from build123d import *

# Parameters (mm, degrees)
BOSS_EXTRUDE1_DEPTH = 30


with BuildPart() as part:
    # Sketch2 → Boss-Extrude1 (new body)
    with BuildSketch(Plane(origin=(0, 0, 0), x_dir=(1, 0, 0), z_dir=(0, 1, 0))):
        with BuildLine():
            Line((0, 90), (-30, 90))
            Line((-30, 90), (-30, 87))
            Line((-30, 87), (0, 87))
            add(Edge.make_bspline(
                [(0, 87), (77.34675255, 84.211391956), (84.31600038, 0)],
                knots=[0, 0, 0, 1, 1, 1], degree=2))
            add(Edge.make_bspline(
                [(0, -87), (77.34675255, -84.211391956), (84.31600038, 0)],
                knots=[0, 0, 0, 1, 1, 1], degree=2))
            Line((0, -87), (-30, -87))
            Line((-30, -87), (-30, -90))
            Line((-30, -90), (0, -90))
            add(Edge.make_bspline(
                [(0, -90), (79.973883015, -87.051000651), (87.31600038, 0)],
                knots=[0, 0, 0, 1, 1, 1], degree=2))
            add(Edge.make_bspline(
                [(0, 90), (79.973883015, 87.051000651), (87.31600038, 0)],
                knots=[0, 0, 0, 1, 1, 1], degree=2))
        make_face()
    extrude(amount=BOSS_EXTRUDE1_DEPTH)


solid = part.part
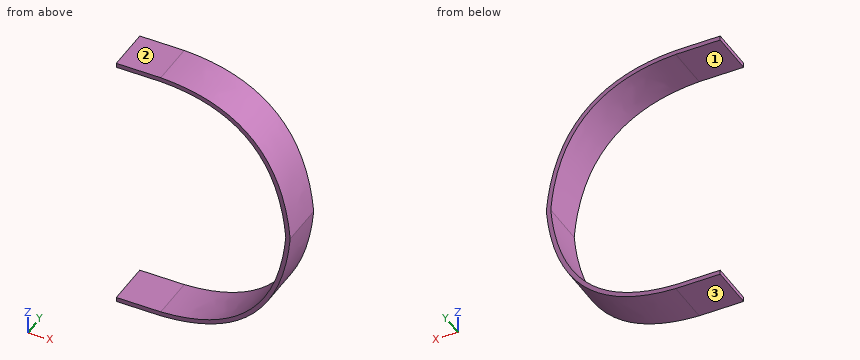
Read the model definition and answer for the solid it produces. Units are mm, in the model's axes. Face numbers are marked on the shaded views. Give positions to 0.01 mm unless a question says otherwise; leave off trailing zeros. Return JSON: item names as keys, results as strings.
Q1. Given P1, Ø10, axis at y = 8, z = 54.5, coming from the -X side; P2, Ø6, axis at x = 41, y = 18, coming from the -Z side; P3, Ø10, axis at y = 26.5, z = 53, coming from the -X side, each flat-ended and moving along its own axis, determine where each tip first touches the part or whether it passes through.
Reply:
{"P1": "x = 63.63", "P2": "z = -82.23", "P3": "x = 64.82"}
Q2. For a pull along Z with two mould halves and no side action, classify the marked faces 1, 2 and 3 as released by +Z, released by -Z, zero draft, split by the parting line, or undercut.
Reply:
{"face 1": "undercut", "face 2": "released by +Z", "face 3": "released by -Z"}
Q3. Consider line 1 along Z through (x, y) = (-11, 5.5); line 2 along Z through (x, y) = (14, 26); line 3 along X through (y, z) = (20, 19.5). Determine where each line is inside the solid, lowest interval first. Write a range as [from, to].
Reply:
{"line 1": "[-90, -87], [87, 90]", "line 2": "[-88.76, -85.74], [85.74, 88.76]", "line 3": "[81.53, 84.55]"}
